from build123d import *

# Parameters (mm, degrees)
F0_W     = 220
F0_H     = 40
F1_DEPTH = 12.5
F2_W     = 41
F2_H     = 10.5
F3_DEPTH = 20
F4_R     = 19.99999
F6_D     = 8.5
F8_D     = 10
F9_R     = 19.99999


# Not quite as in the source:
# - a fillet or chamfer is up to 0.001 mm smaller than in the source, because OpenCascade refuses the exact size


with BuildPart() as f1:
    # F0 (on Top) → F1 (new body, symmetric)
    with BuildSketch(Plane.XY):
        Rectangle(F0_W, F0_H)
    extrude(amount=F1_DEPTH, both=True)

    # F2 (on Front) → F3 (cut, symmetric)
    with BuildSketch(Plane.XZ):
        with Locations((-89.5, 0)):
            Rectangle(F2_W, F2_H)
    extrude(amount=F3_DEPTH, both=True, mode=Mode.SUBTRACT)

    # F4 (radius 20 in the source; OpenCascade refuses exactly that, so slightly less here)
    f4_edges = [f1.edges().sort_by_distance(p)[0] for p in [
        (-110, 20, 8.875),
        (-110, -20, 8.875),
        (-110, -20, -8.875),
        (-110, 20, -8.875),
    ]]
    fillet(f4_edges, radius=F4_R)

    # F6 (through all)
    with Locations(Plane(origin=(0, 0, -12.5), x_dir=(1, 0, 0), z_dir=(0, 0, -1))):
        with Locations((-90, 0)):
            Hole(F6_D / 2)

    # F8 (through all)
    with Locations(Plane(origin=(0, 0, -12.5), x_dir=(1, 0, 0), z_dir=(0, 0, -1))):
        with Locations((90, 0)):
            Hole(F8_D / 2)

    # F9 (radius 20 in the source; OpenCascade refuses exactly that, so slightly less here)
    f9_edges = [f1.edges().sort_by_distance(p)[0] for p in [
        (110, -20, 0),
        (110, 20, 0),
    ]]
    fillet(f9_edges, radius=F9_R)


solid = f1.part
Verification items for the finished model (mm, model axes). A direction names the side the tool comes from. Give positions to 0.01 mm unless a question says otherwise; leave off trailing zeros. Order: outer loops, then holes, each group sorted by start corner. A loop starts at its lowest first (then second) coordinate and runs counter-clockwise, first axis right, second up. Notation, with made-up numbers: (12.5, 30) -> (61.5, 30) arc R24 ccw to (61.5, 57) -> close; hole circle Ø4 at (32, 0.5). An arc over 180 degrees is marked (long way). Answer as CSV lines item,"result".
Q1. Sectioned sample at C-C on y = -12. Record the cut outline in (x, z).
Solutions:
outline,"(-106, -12.5) -> (106, -12.5) -> (106, 12.5) -> (-106, 12.5) -> (-106, 5.25) -> (-69, 5.25) -> (-69, -5.25) -> (-106, -5.25) -> close"
Q2. Sectioned sample at A-A on x = -78. Record the cut outline in (y, z), plus the area to 3 significant figures.
Solutions:
outline,"(-20, -12.5) -> (20, -12.5) -> (20, -5.25) -> (-20, -5.25) -> close; (-20, 5.25) -> (20, 5.25) -> (20, 12.5) -> (-20, 12.5) -> close"
area,"580 mm²"
Q3. Sectioned sample at B-B on z = 8.25. Count the separate pieces of the cut face and the enclosed holes in it, plus the area to 3 significant figures.
Solutions:
separate pieces,"1"
enclosed holes,"2"
area,"8,320 mm²"
Q4. Depth check by flat-ended pin: pin 1 (1.5 mm diameter, centred on y = 15.5, z = 2, fed in from +X); pin 2 (5 mm diameter, centred on y = -10, z = -2, fed in from -X). Enter the tip coordinate at first touch or a pass-through.
Solutions:
pin 1,"stops at x = 103.51"
pin 2,"stops at x = -69"
Q5. Release check for a two-part mould opening along X. For faces 3 (the cylindrical face through (-85.754, -0.187, -8.824)), 4 (the cylindrical face through (103.986, 14.297, -0.175)), 5 (the cylindrical face through (-103.986, 14.297, 8.824)) record: +X half, -X half, draft (parallel to the pull), parting line (faces both ways), or undercut.
Solutions:
face 3,"undercut"
face 4,"+X half"
face 5,"-X half"
Q6. Access from +Z, -Z, +X, -X, +Y, -Y to the whole of each face (thin tool, end or side, straight path). Record for faces 1 (the flat face through (-85, 0, -5.25)), 2 (the flat face through (-2, 0, 12.5)).
Solutions:
face 1,"-X, +Y, -Y"
face 2,"+Z, +X, -X, +Y, -Y"
Q7. Scan lines: probe 1 along X at (y, z) = (-2.5, 6); probe 2 along Y at (x, z) = (-90, 8.25); probe 3 along Z at (x, y) = (-83, 8.5). Record each from-to range of solid material in increasing order.
Solutions:
probe 1,"x = -109.84 to -93.44, -86.56 to 85.67, 94.33 to 109.84"
probe 2,"y = -20 to -4.25, 4.25 to 20"
probe 3,"z = -12.5 to -5.25, 5.25 to 12.5"
